Part model, mm, in its own coordinate system. Give positions to 0.01 mm unless a question says otherwise; leave off trailing zeros. Order: outer loops, then holes, each group sorted by start corner. A loop starts at its lowest first (then second) coordinate and runs counter-clockwise, first axis right, second up.
from build123d import *

# Parameters (mm, degrees)
F0_W     = 45
F0_H     = 45
F0_R     = 4.5
F1_DEPTH = 500
F3_D     = 6
F3_DEPTH = 4
F3_TIP   = 1.8025818571


with BuildPart() as f1:
    # F0 (on Right) → F1 (new body)
    with BuildSketch(Plane.YZ):
        Rectangle(F0_W, F0_H)
        Circle(F0_R, mode=Mode.SUBTRACT)
    extrude(amount=-F1_DEPTH)

    # F3
    with Locations(Plane(origin=(0, 0, -22.5), x_dir=(1, 0, 0), z_dir=(0, 0, -1))):
        with Locations((-50, 0), (-450, 0)):
            Hole(F3_D / 2, depth=F3_DEPTH)
            with Locations((0, 0, -(F3_DEPTH + F3_TIP / 2))):  # 118° drill point
                Cone(0, F3_D / 2, F3_TIP, mode=Mode.SUBTRACT)


solid = f1.part
Item 1: Band-saw the part on B-B on x = -382. List the corners of the cut face in (y, z), plus the area to 3 significant figures.
Item 2: Drill centre lines: probe 1 along Y at (x, z) = (-50, -21.65); probe 2 along Y at (x, z) = (-478.5, -2); probe 3 along Z at (x, y) = (-57, 3.5). Where is each one in solid material? Low to high.
Item 3: Drop a flat-ended pin along its axis: P1, Ø7, axis at x = -450, y = 0, coming from the -Z side. Give the stop position or say it passes through.
Item 4: Pull direction Y, two halves, no side cores. Call faces 1 (the face through (-246, 0, 22.5)), 2 (the face through (-246.5, -0.59, 4.46)), 3 (the face through (-246, -22.5, 0)): released by +Y, released by -Y, zero draft, split by the parting line, or undercut.
Item 5: Band-saw the part on A-A on z = 0. List the corners of the cut face in (x, y).
Working result:
1. outline: (-22.5, -22.5) - (22.5, -22.5) - (22.5, 22.5) - (-22.5, 22.5) - close; hole circle Ø9 at (0, 0)
1. area: 1,960 mm2
2. probe 1: y = -22.5 to -3, 3 to 22.5
2. probe 2: y = -22.5 to -4.03, 4.03 to 22.5
2. probe 3: z = -22.5 to -2.83, 2.83 to 22.5
3. P1: stops at z = -22.5
4. face 1: zero draft
4. face 2: undercut
4. face 3: released by -Y
5. outline: (-500, -22.5) - (0, -22.5) - (0, -4.5) - (-500, -4.5) - close; (-500, 4.5) - (0, 4.5) - (0, 22.5) - (-500, 22.5) - close
